The model under review builds one solid part; all positions refer to its coordinate system, in mm. Round coordinates to 2 decimals unless told otherwise and drop trailing zeros. Write each loop counter-clockwise with the first axis right and the second up, starting at its lowest first coordinate (ties: lowest second). Pieces come first, ordered by that corner, then holes.
Item 1: To check wall thickness, follow L1, parallel to X at y = 831, z = -13.25; L2, parallel to Z at x = 6.5, y = 1000.5; L3, parallel to Z at x = 2.5, y = 722.5. State the ranges of each line that lie inside material, in increasing order.
Item 2: Clearance check with flat-ended pins moving along their axes: pin 1 Ø1.2 at (x, y) = (0.5, 488) entering from -Z; pin 2 Ø1.6 at (y, z) = (8, -1) entering from +X; pin 3 Ø0.8 at (x, y) = (0.5, 727) entering from -Z. State where each tip first meets the part, or that it passes through.
Item 3: Add section B-B (z = -12). State how many separate pieces and enclosed holes the cut face has, plus the area to 3 significant figures.
Item 4: Add section A-A (y = 291). Give the boundary of the cut face in (x, z), plus the area to 3 significant figures.
```python
from build123d import *

# Parameters (mm, degrees)
SKETCH1_W                   = 17
SKETCH1_H                   = 17
BOSS_EXTRUDE1_DEPTH         = 1220
SKETCH2_W                   = 20
SKETCH2_H                   = 20
CUT_EXTRUDE1_DEPTH          = 10
CUT_EXTRUDE2_DEPTH          = 15
SKETCH4_W                   = 3
SKETCH4_H                   = 10
CUT_EXTRUDE3_DEPTH          = 10
SKETCH_PATTERN1_START       = -20
SKETCH_PATTERN1_DEPTH       = 15
SKETCH_PATTERN1_2_OUTLINE_W = 1.5
SKETCH_PATTERN1_2_OUTLINE_H = 10
SKETCH_PATTERN1_2_DEPTH     = 3
SKETCH6_W                   = 20
SKETCH6_H                   = 20
CUT_EXTRUDE4_DEPTH          = 4
SKETCH7_W                   = 11
SKETCH7_H                   = 5
CUT_EXTRUDE5_DEPTH          = 1221.327824808
LPATTERN1_COUNT             = 2
LPATTERN1_PITCH             = 400


# Read off the part's stored shape, not the designer's step: Sketch-Pattern1
with BuildPart() as part:
    # Sketch1 → Boss-Extrude1 (new body)
    with BuildSketch(Plane(origin=(0, 0, 0), x_dir=(1, 0, 0), z_dir=(0, 1, 0))):
        with BuildLine():
            Line((0.5, 0), (19.5, 0))
            ThreePointArc((19.5, 0), (19.853553391, 0.146446609), (20, 0.5))
            Line((20, 0.5), (20, 19.5))
            ThreePointArc((20, 19.5), (19.853553391, 19.853553391), (19.5, 20))
            Line((19.5, 20), (0.5, 20))
            ThreePointArc((0.5, 20), (0.146446609, 19.853553391), (0, 19.5))
            Line((0, 19.5), (0, 0.5))
            ThreePointArc((0, 0.5), (0.146446609, 0.146446609), (0.5, 0))
        make_face()
        with Locations((10, 10)):
            Rectangle(SKETCH1_W, SKETCH1_H, mode=Mode.SUBTRACT)
    extrude(amount=BOSS_EXTRUDE1_DEPTH)

    # Sketch2 → Cut-Extrude1 (cut)
    with BuildSketch(Plane(origin=(20, 0, 0), x_dir=(0, 0, -1), z_dir=(1, 0, 0))):
        with Locations((10, 1210)):
            Rectangle(SKETCH2_W, SKETCH2_H)
        with Locations((10, 10)):
            Rectangle(SKETCH2_W, SKETCH2_H)
    extrude(amount=-CUT_EXTRUDE1_DEPTH, mode=Mode.SUBTRACT)

    # Sketch3 → Cut-Extrude2 (cut)
    with BuildSketch(Plane(origin=(0, 0, -20), x_dir=(-1, 0, 0), z_dir=(0, 0, -1))):
        Polygon((-15, 1115), (0, 1115), (0, 1120), (-9, 1120), (-9, 1130), (0, 1130), (0, 1135), (-15, 1135), align=None)
    extrude(amount=-CUT_EXTRUDE2_DEPTH, mode=Mode.SUBTRACT)

    # Sketch4 → Cut-Extrude3 (cut)
    with BuildSketch(Plane.ZY):
        with Locations((-18.5, 1125)):
            Rectangle(SKETCH4_W, SKETCH4_H)
    extrude(amount=-CUT_EXTRUDE3_DEPTH, mode=Mode.SUBTRACT)

    # Sketch-Pattern1 outline → Sketch-Pattern1 (cut)
    with BuildSketch(Plane.XY.offset(SKETCH_PATTERN1_START)):
        Polygon((15, 85), (15, 105), (0, 105), (0, 100), (1.5, 100), (1.5, 90), (0, 90), (0, 85), align=None)
        Polygon((1.5, 330), (1.5, 320), (0, 320), (0, 315), (15, 315), (15, 335), (0, 335), (0, 330), align=None)
        Polygon((1.5, 500), (1.5, 490), (0, 490), (0, 485), (15, 485), (15, 505), (0, 505), (0, 500), align=None)
        Polygon((1.5, 730), (1.5, 720), (0, 720), (0, 715), (15, 715), (15, 735), (0, 735), (0, 730), align=None)
        Polygon((1.5, 900), (1.5, 890), (0, 890), (0, 885), (15, 885), (15, 905), (0, 905), (0, 900), align=None)
    extrude(amount=SKETCH_PATTERN1_DEPTH, mode=Mode.SUBTRACT)

    # Sketch-Pattern1 2 outline → Sketch-Pattern1 2 (cut)
    with BuildSketch(Plane.XY.offset(SKETCH_PATTERN1_START)):
        with Locations((0.75, 95)):
            Rectangle(SKETCH_PATTERN1_2_OUTLINE_W, SKETCH_PATTERN1_2_OUTLINE_H)
        with Locations((0.75, 325)):
            Rectangle(SKETCH_PATTERN1_2_OUTLINE_W, SKETCH_PATTERN1_2_OUTLINE_H)
        with Locations((0.75, 495)):
            Rectangle(SKETCH_PATTERN1_2_OUTLINE_W, SKETCH_PATTERN1_2_OUTLINE_H)
        with Locations((0.75, 725)):
            Rectangle(SKETCH_PATTERN1_2_OUTLINE_W, SKETCH_PATTERN1_2_OUTLINE_H)
        with Locations((0.75, 895)):
            Rectangle(SKETCH_PATTERN1_2_OUTLINE_W, SKETCH_PATTERN1_2_OUTLINE_H)
    extrude(amount=SKETCH_PATTERN1_2_DEPTH, mode=Mode.SUBTRACT)

    # Sketch6 → Cut-Extrude4 (cut)
    with BuildSketch(Plane(origin=(20, 0, 0), x_dir=(0, 0, -1), z_dir=(1, 0, 0))):
        with Locations((10, 810)):
            Rectangle(SKETCH6_W, SKETCH6_H)
    cut_extrude4 = extrude(amount=-CUT_EXTRUDE4_DEPTH, mode=Mode.SUBTRACT)

    # Sketch7 → Cut-Extrude5 (cut, symmetric)
    with BuildSketch(Plane(origin=(0, 0, -20), x_dir=(-1, 0, 0), z_dir=(0, 0, -1))):
        with Locations((-10.5, 817.5)):
            Rectangle(SKETCH7_W, SKETCH7_H)
        with Locations((-10.5, 802.5)):
            Rectangle(SKETCH7_W, SKETCH7_H)
    cut_extrude5 = extrude(amount=CUT_EXTRUDE5_DEPTH, both=True, mode=Mode.SUBTRACT)

    # LPattern1: Cut-Extrude4, Cut-Extrude5 ×2
    with Locations(*[(0, -i * LPATTERN1_PITCH, 0) for i in range(1, LPATTERN1_COUNT)]):
        add(cut_extrude4, mode=Mode.SUBTRACT)
        add(cut_extrude5, mode=Mode.SUBTRACT)


solid = part.part
```
Numbers:
1. L1: x = 0 to 1.5, 18.5 to 20
1. L2: z = -20 to -18.5, -1.5 to 0
1. L3: z = -1.5 to 0
2. pin 1: stops at z = -5
2. pin 2: stops at x = 10
2. pin 3: stops at z = -17
3. separate pieces: 16
3. enclosed holes: 0
3. area: 3,450 mm2
4. outline: (0, -19.5) arc R0.5 ccw to (0.5, -20) - (19.5, -20) arc R0.5 ccw to (20, -19.5) - (20, -0.5) arc R0.5 ccw to (19.5, 0) - (0.5, 0) arc R0.5 ccw to (0, -0.5) - close; hole (1.5, -18.5) - (18.5, -18.5) - (18.5, -1.5) - (1.5, -1.5) - close
4. area: 111 mm2
